Build history of the part. All positions in model axes, mm. Face numbers are marked on the shaded views. Give positions to 0.01 mm unless a question says otherwise; leave off trailing zeros. Loops run counter-clockwise (first coordinate to the right, second up) from the corner with the lowest first, then second, coordinate; pieces in that order, holes last. Notation, with made-up numbers: M -5,45 L 23,45 A12 cw 23,68 Z; hole C -8.75,40.25 d9. An arc over 180 degrees is marked long. Put each result on its own line as item: value.
Autodesk Inventor part; units mm, degrees
ref_plane "YZ Plane" through (0, 0, 0) normal (1, 0, 0) x (0, 1, 0)
ref_plane "XZ Plane" through (0, 0, 0) normal (0, 1, 0) x (-1, 0, 0)
ref_plane "XY Plane" through (0, 0, 0) normal (0, 0, 1) x (1, 0, 0)
sketch "Boceto1" plane through (0, 0, 0) normal (0, 1, 0) x (-1, 0, 0)
  line L0 (-3, -10) -> (3, -10)
  line L1 (3, -10) -> (3, 10)
  line L2 (3, 10) -> (-3, 10)
  line L3 (-3, 10) -> (-3, -10)
  line L4 (-3, -10) -> (3, 10) construction
  line L5 (3, -10) -> (-3, 10) construction
  point P0 (0, 0)
  dimension "d0" = 6
  dimension "d1" = 20
extrude "Extrusión1" add sketch "Boceto1" along normal blind 4
sketch "Boceto2" plane through (-3, 0, -10) normal (-1, 0, 0) x (0, 0, 1)
  line L0 (0, 0) -> (0, 4)
  line L1 (0, 4) -> (3.3564, 0)
  line L2 (0, 0) -> (20, 0)
  line L3 (0, 4) -> (5.2216, 4) construction
  line L4 (3.3564, 0) -> (0, 0)
  line L5 (0, 0) -> (0, 4)
  line L6 (20, 0) -> (16.6436, 4)
  line L7 (0, 4) -> (20, 4)
  line L8 (20, 0) -> (25.2216, 0) construction
  line L9 (16.6436, 4) -> (12.8134, 0.7861)
  line L10 (12.8134, 0.7861) -> (19.2413, -6.8744)
  line L11 (19.2413, -6.8744) -> (23.0715, -3.6604)
  line L12 (23.0715, -3.6604) -> (20, 0)
  line L13 (20, 4) -> (23.0715, -3.6604)
  line L14 (20, 4) -> (16.6436, 4)
  line L15 (13.473, 0) -> (15.4013, -2.2981)
  line L16 (15.4013, -2.2981) -> (13.1032, -4.2265)
  line L17 (13.1032, -4.2265) -> (13.1032, 0)
  point P0 (10, 0)
  point P1 (14.7285, 2.393)
  point P2 (14.8694, 0)
  point P3 (11.8766, 0)
  dimension "d9" = 50
  dimension "d10" = 130
  dimension "d11" = 90
  dimension "d12" = 10
  dimension "d15" = 5
  dimension "d16" = 3
  dimension "d17" = 3
draft "Cara para el ángulo de desmoldeo1" angle 10 pull direction (0, 1, 0) faces at (3, 2.6667, 3.3333) fixed edges at (3, 4, 0)
mirror "Simetría1" about plane through (0, 0, 0) normal (1, 0, 0) of "Extrusión1", "Cara para el ángulo de desmoldeo1"
extrude "Extrusión2" cut sketch "Boceto2" along normal mid plane 20 contours L0 L1 L2
extrude "Extrusión3" add sketch "Boceto2" along normal blind 0.7 and the other way blind 6.7 contours L7 L13 L12 L6 | L6 L2 L10 L9 | L2 L10 L16 L17 | L12 L11 L10 L2
chamfer "Chaflán1" distance 2 angle 45 1 edges at (0, 0, 3.1032)
fillet "Empalme1" radius 0.2 1 edges at (0, -4.2265, 3.1032)
properties part number "palitowantan"
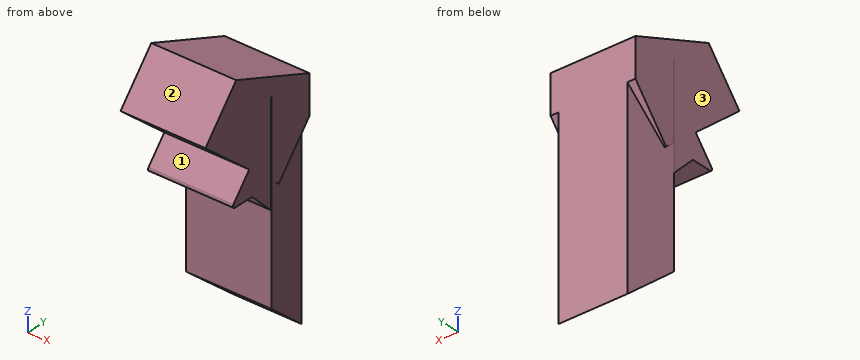
Q1. Slice it at B-B (z = -0.75). List the corners of the cut face in (x, y), and give its area (3 significant figures).
Here are the results:
outline: M -3.71,0 L 3.71,0 L 3,4 L -3,4 Z
area: 26.8 mm²
Q2. Slice it at A-A (x = -1.5). List the corners of the cut face in (y, z), and give its area (3 significant figures).
Here are the results:
outline: M -6.87,9.24 L -2.3,5.4 L -3.95,3.43 A0.2 ccw -3.8,3.1 L -2,3.1 L 0,1.1 L 0,-6.64 L 4,-10 L 4,10 L -3.66,13.07 Z
area: 121 mm²
Q3. Drop flat-ended pins along their axis: pin 1 Ø6 at (y, z) = (1, 2.5) entering from -X; pin 2 Ø1 at (y, z) = (-1, 6.5) entering from +X; pin 3 Ø0.9 at (x, y) = (-0.5, -2.5) entering from -Z. Give the stop position or say it passes through.
Here are the results:
pin 1: x = -3.71
pin 2: x = 3.7
pin 3: z = 3.1
Q4. Probe line 1 (Y direction, x = 1, z = -6); line 2 (Z direction, x = -1.25, y = -3.25); line 3 (X direction, y = 3.75, z = 7.75). List the from-to ranges inside material, lowest first. Write a range as from..to.
Here are the results:
line 1: 0..4
line 2: 3.1..4.27, 6.2..12.91
line 3: -3.7..3.7
Q5. Mould opens along Z. For the marked faces 1, 2 and 3 say: pulls with the +Z half, pulls with the -Z half, needs draft (parallel to the pull), parting line crosses it, or undercut.
Here are the results:
face 1: undercut
face 2: pulls with the +Z half
face 3: needs draft
Q6. Slice it at C-C (y = -5.5). List the corners of the cut face in (x, z).
Here are the results:
outline: M -3.7,8.09 L 3.7,8.09 L 3.7,10.88 L -3.7,10.88 Z
